Part model, mm, in its own coordinate system. Face numbers are marked on the shaded views. A direction names the side the tool comes from. Coordinates: 2 decimals unless noted, no trailing zeros. Write each loop counter-clockwise with the first axis right and the second up, starting at its lowest first coordinate (ties: lowest second). Pieces come first, ordered by that corner, then holes. Notation, with made-up numbers: (34.25, 54.25) -> (47.25, 54.25) arc R24 ccw to (47.25, 87.25) -> close; hole circle Ø3 at (-7, 27). An arc over 180 degrees is marked (long way). Write item = value, one per line. Start each with the question number.
Q1. Pull direction Y, two halves, no side cores. Call the marked faces 3, 4 and 5: released by +Y, released by -Y, zero draft, split by the parting line, or undercut.
Q2. Tool access for the marked faces 1 and 2: list every direction of +Z, -Z, +X, -X, +Y, -Y with a clear straight run to the whole face (end or side of a thin tool).
Q3. Probe line 1 (Y direction, x = 1.5, z = -2.5); line 2 (X direction, y = 26, z = 3); line 3 (X direction, y = 31.5, z = 2.5). List the from-to ranges inside material, lowest first.
Q4. Pin check, flat tips, straight feed: P1, Ø1, axis at y = -0.5, z = 1.5, coming from the +X side; P2, Ø3, axis at x = 45, z = 0, coming from the -Y side; P3, Ø8, axis at x = 40.5, y = 31.5, coming from the +Z side (3 decimals); P4, Ø3, axis at x = 35.5, z = 4, coming from the +Y side. Stop position of each tip, or through.
Q5. Band-saw the part on A-A, the plane x = 20.5. List the corners of the cut face in (y, z) (3 decimals), plus the area to 3 significant figures.
Q6. Band-saw the part on C-C, the plane x = -68.5. List the corners of the cut face in (y, z) (3 decimals), plus the area to 3 significant figures.
Q7. Band-saw the part on B-B, the plane y = 48.5. List the corners of the cut face in (x, z) (3 decimals), plus the area to 3 significant figures.
from build123d import *

# Parameters (mm, degrees)
F0_R          = 88.9
F1_DEPTH      = 6.35
F1_DEPTH_BACK = 6.35
F2_DEPTH      = 3.175
F2_DEPTH_BACK = 3.175
F3_W          = 3.175
F3_H          = 3.175
F4_DEPTH      = 127
F4_DEPTH_BACK = 25.4


with BuildPart() as f1:
    # F0 (on Top) → F1 (new body, two sides)
    with BuildSketch(Plane.XY) as f1_sk:
        Circle(F0_R)
        with BuildLine():
            ThreePointArc((76.0304780992, 5.08), (76.1576077328, 2.5414138621), (76.2, 0))
            ThreePointArc((76.2, 0), (76.1576077328, -2.5414138621), (76.0304780992, -5.08))
            ThreePointArc((76.0304780992, -5.08), (70.1110952475, -29.8475178733), (56.3616350551, -51.2816350551))
            ThreePointArc((56.3616350551, -51.2816350551), (53.8815367264, -53.8815367264), (51.2816350551, -56.3616350551))
            ThreePointArc((51.2816350551, -56.3616350551), (29.8475178733, -70.1110952475), (5.08, -76.0304780992))
            ThreePointArc((5.08, -76.0304780992), (0, -76.2), (-5.08, -76.0304780992))
            ThreePointArc((-5.08, -76.0304780992), (-29.8475178733, -70.1110952475), (-51.2816350551, -56.3616350551))
            ThreePointArc((-51.2816350551, -56.3616350551), (-53.8815367264, -53.8815367264), (-56.3616350551, -51.2816350551))
            ThreePointArc((-56.3616350551, -51.2816350551), (-70.1110952475, -29.8475178733), (-76.0304780992, -5.08))
            ThreePointArc((-76.0304780992, -5.08), (-76.2, 0), (-76.0304780992, 5.08))
            ThreePointArc((-76.0304780992, 5.08), (-70.1110952475, 29.8475178733), (-56.3616350551, 51.2816350551))
            ThreePointArc((-56.3616350551, 51.2816350551), (-53.8815367264, 53.8815367264), (-51.2816350551, 56.3616350551))
            ThreePointArc((-51.2816350551, 56.3616350551), (-29.8475178733, 70.1110952475), (-5.08, 76.0304780992))
            ThreePointArc((-5.08, 76.0304780992), (0, 76.2), (5.08, 76.0304780992))
            ThreePointArc((5.08, 76.0304780992), (29.8475178733, 70.1110952475), (51.2816350551, 56.3616350551))
            ThreePointArc((51.2816350551, 56.3616350551), (53.8815367264, 53.8815367264), (56.3616350551, 51.2816350551))
            ThreePointArc((56.3616350551, 51.2816350551), (70.1110952475, 29.8475178733), (76.0304780992, 5.08))
        make_face(mode=Mode.SUBTRACT)
    extrude(amount=F1_DEPTH)
    extrude(f1_sk.sketch, amount=-F1_DEPTH_BACK)

    # F0 (on Top) → F2 (join, two sides)
    with BuildSketch(Plane.XY) as f2_sk:
        with BuildLine():
            ThreePointArc((76.0304780992, -5.08), (76.1576077328, -2.5414138621), (76.2, 0))
            ThreePointArc((76.2, 0), (76.1576077328, 2.5414138621), (76.0304780992, 5.08))
            Line((76.0304780992, 5.08), (10.16, 5.08))
            Line((10.16, 5.08), (56.3616350551, 51.2816350551))
            ThreePointArc((56.3616350551, 51.2816350551), (53.8815367264, 53.8815367264), (51.2816350551, 56.3616350551))
            Line((51.2816350551, 56.3616350551), (5.08, 10.16))
            Line((5.08, 10.16), (5.08, 76.0304780992))
            ThreePointArc((5.08, 76.0304780992), (0, 76.2), (-5.08, 76.0304780992))
            Line((-5.08, 76.0304780992), (-5.08, 10.16))
            Line((-5.08, 10.16), (-51.2816350551, 56.3616350551))
            ThreePointArc((-51.2816350551, 56.3616350551), (-53.8815367264, 53.8815367264), (-56.3616350551, 51.2816350551))
            Line((-56.3616350551, 51.2816350551), (-10.16, 5.08))
            Line((-10.16, 5.08), (-76.0304780992, 5.08))
            ThreePointArc((-76.0304780992, 5.08), (-76.2, 0), (-76.0304780992, -5.08))
            Line((-76.0304780992, -5.08), (-10.16, -5.08))
            Line((-10.16, -5.08), (-56.3616350551, -51.2816350551))
            ThreePointArc((-56.3616350551, -51.2816350551), (-53.8815367264, -53.8815367264), (-51.2816350551, -56.3616350551))
            Line((-51.2816350551, -56.3616350551), (-5.08, -10.16))
            Line((-5.08, -10.16), (-5.08, -76.0304780992))
            ThreePointArc((-5.08, -76.0304780992), (0, -76.2), (5.08, -76.0304780992))
            Line((5.08, -76.0304780992), (5.08, -10.16))
            Line((5.08, -10.16), (51.2816350551, -56.3616350551))
            ThreePointArc((51.2816350551, -56.3616350551), (53.8815367264, -53.8815367264), (56.3616350551, -51.2816350551))
            Line((56.3616350551, -51.2816350551), (10.16, -5.08))
            Line((10.16, -5.08), (76.0304780992, -5.08))
        make_face()
    extrude(amount=F2_DEPTH)
    extrude(f2_sk.sketch, amount=-F2_DEPTH_BACK)

    # F3 (on face) → F4 (cut, two sides)
    with BuildSketch(Plane.XY) as f4_sk:
        Rectangle(F3_W, F3_H)
    extrude(amount=-F4_DEPTH, mode=Mode.SUBTRACT)
    extrude(f4_sk.sketch, amount=F4_DEPTH_BACK, mode=Mode.SUBTRACT)


solid = f1.part
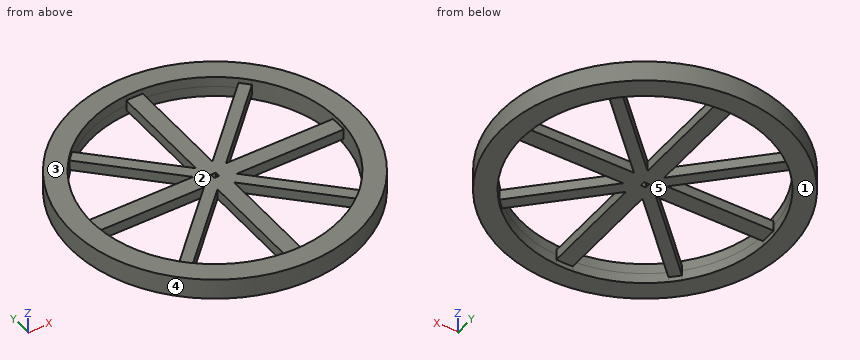
Ans:
q1.face_3 = zero draft
q1.face_4 = split by the parting line
q1.face_5 = undercut
q2.face_1 = -Z, +X, -X, +Y, -Y
q2.face_2 = +Z
q3.line_1 = -88.89 to -1.59, 1.59 to 88.89
q3.line_2 = -85.01 to -71.63, -31.08 to -20.92, -5.08 to 5.08, 20.92 to 31.08, 71.63 to 85.01
q3.line_3 = -83.13 to -69.38, -36.58 to -26.42, -5.08 to 5.08, 26.42 to 36.58, 69.38 to 83.13
q4.P1 = 88.9
q4.P2 = -77.53
q4.P3 = 3.175
q4.P4 = 82.14
q5.outline = (-86.504, -6.35) -> (-73.391, -6.35) -> (-73.391, 6.35) -> (-86.504, 6.35) -> close; (-25.58, -3.175) -> (-15.42, -3.175) -> (-15.42, 3.175) -> (-25.58, 3.175) -> close; (-5.08, -3.175) -> (5.08, -3.175) -> (5.08, 3.175) -> (-5.08, 3.175) -> close; (15.42, -3.175) -> (25.58, -3.175) -> (25.58, 3.175) -> (15.42, 3.175) -> close; (73.391, -6.35) -> (86.504, -6.35) -> (86.504, 6.35) -> (73.391, 6.35) -> close
q5.area = 527 mm2
q6.outline = (-56.665, -6.35) -> (-33.379, -6.35) -> (-33.379, 6.35) -> (-56.665, 6.35) -> close; (-5.08, -3.175) -> (5.08, -3.175) -> (5.08, 3.175) -> (-5.08, 3.175) -> close; (33.379, -6.35) -> (56.665, -6.35) -> (56.665, 6.35) -> (33.379, 6.35) -> close
q6.area = 656 mm2
q7.outline = (-74.505, -6.35) -> (-58.772, -6.35) -> (-58.772, 6.35) -> (-74.505, 6.35) -> close; (-53.58, -3.175) -> (-43.42, -3.175) -> (-43.42, 3.175) -> (-53.58, 3.175) -> close; (-5.08, -3.175) -> (5.08, -3.175) -> (5.08, 3.175) -> (-5.08, 3.175) -> close; (43.42, -3.175) -> (53.58, -3.175) -> (53.58, 3.175) -> (43.42, 3.175) -> close; (58.772, -6.35) -> (74.505, -6.35) -> (74.505, 6.35) -> (58.772, 6.35) -> close
q7.area = 593 mm2
